from build123d import *

# Parameters (mm, degrees)
PAD_DEPTH       = 27.5
PAD_DEPTH_BACK  = 27.5
FILLET_R        = 2
SKETCH001_W     = 52
SKETCH001_H     = 11.986657
POCKET_DEPTH    = 30
SKETCH002_R     = 1.65
POCKET001_DEPTH = 14.114999
SKETCH003_R     = 1.65
POCKET002_DEPTH = 2.001
FILLET001_R     = 2.5


with BuildPart() as part:
    # Sketch → Pad (new body, two sides)
    with BuildSketch(Plane.YZ) as pad_sk:
        Polygon((0, 0), (15, 0), (0, 40), align=None)
    extrude(amount=PAD_DEPTH)
    extrude(pad_sk.sketch, amount=-PAD_DEPTH_BACK)

    # Fillet
    fillet_edges = [part.edges().sort_by_distance(p)[0] for p in [
        (0, 0, 40),
        (0, 15, 0),
    ]]
    fillet(fillet_edges, radius=FILLET_R)

    # Sketch001 (on DatumPlane) → Pocket (cut)
    with BuildSketch(Plane.XY.offset(32)):
        with Locations((0, 7.993328)):
            Rectangle(SKETCH001_W, SKETCH001_H)
    extrude(amount=-POCKET_DEPTH, mode=Mode.SUBTRACT)

    # Sketch002 (on Face4 of Pocket) → Pocket001 (cut, through all)
    with BuildSketch(Plane(origin=(0, 0, 0), x_dir=(0, 0, -1), z_dir=(0, -1, 0))):
        with Locations((-14.485332, 22.5)):
            Circle(SKETCH002_R)
        with Locations((-14.485332, -22.5)):
            Circle(SKETCH002_R)
    extrude(amount=-POCKET001_DEPTH, mode=Mode.SUBTRACT)

    # Sketch003 (on Face15 of Pocket001) → Pocket002 (cut, through all)
    with BuildSketch(Plane(origin=(0, 0, 2), x_dir=(0, -1, 0), z_dir=(0, 0, 1))):
        with Locations((-7.986657, 15)):
            Circle(SKETCH003_R)
        with Locations((-7.986657, -15)):
            Circle(SKETCH003_R)
    extrude(amount=-POCKET002_DEPTH, mode=Mode.SUBTRACT)

    # Fillet001
    fillet001_edges = [part.edges().sort_by_distance(p)[0] for p in [
        (0, 2, 2),
    ]]
    fillet(fillet001_edges, radius=FILLET001_R)


solid = part.part
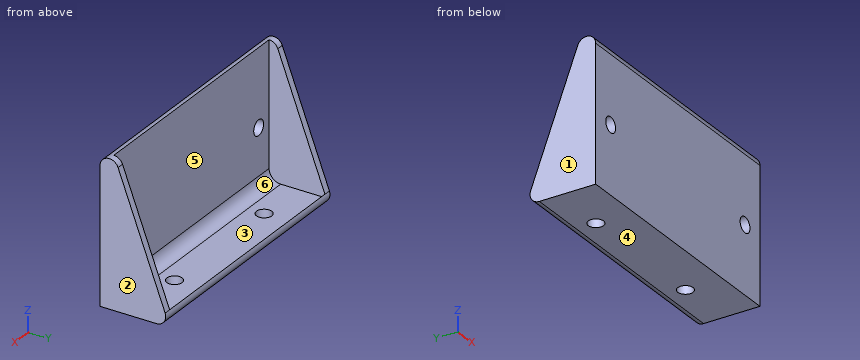
Can you work these out from the model? Positions are in its coordinate system, mm. Face numbers are marked on the shaded views. A direction names the side the tool comes from. Round coordinates to 2 decimals unless told otherwise and drop trailing zeros. Loops run counter-clockwise (first coordinate to the right, second up) from the corner with the lowest first, then second, coordinate; pieces in that order, holes last. Notation, with made-up numbers: (65.5, 7.25) - (115.5, 7.25) arc R26 cw to (115.5, 41.25) - close; hole circle Ø9 at (67, 28). An arc over 180 degrees is marked (long way). Use CSV: the item, a comma, the result in double quotes. Start each with the question number.
1) We'd pull the mould along X, two halves only. Please class the marked faces 1, 2 and 3: released by +X, released by -X, zero draft, split by the parting line, or undercut.
2) If we section it at B-B on y = 8.25: Write out the boundary of the cut face in (x, z).
3) For pin 1 Ø8 at (x, z) = (-7, 16) entering from +Y; pin 2 Ø3 at (x, z) = (22.5, 14.49) entering from -Y; pin 3 Ø1 at (x, y) = (-21, 11) entering from +Z; pin 4 Ø7.5 at (x, y) = (13, 7.5) entering from +Z, each with a flat end and sliding along its axis, tell me the tip position at first contact or that it passes through.
4) For the marked faces 4, 5 and 6, which set-ups out of +Z, -Z, +X, -X, +Y, -Y let a thin tool reach every point of the face, with its end or its side?
5) If we section it at C-C on z = 7: Write out the boundary of the cut face in (x, y) (3 decimals).
6) Please list where these lines run through material, in increasing order: probe 1 along X at (y, z) = (5.75, 15.5); probe 2 along Z at (x, y) = (-23.5, 6). Write a range as [from, to].
Geometry results:
1,face 1,"released by -X"
1,face 2,"released by +X"
1,face 3,"undercut"
2,outline,"(-27.5, 0) - (-16.63, 0) - (-16.63, 2) - (-26, 2) - (-26, 18) - (-27.5, 18) - close; (-13.37, 0) - (13.37, 0) - (13.37, 2) - (-13.37, 2) - close; (16.63, 0) - (27.5, 0) - (27.5, 18) - (26, 18) - (26, 2) - (16.63, 2) - close"
3,pin 1,"stops at y = 2"
3,pin 2,"passes through"
3,pin 3,"stops at z = 2"
3,pin 4,"stops at z = 2.12"
4,face 4,"-Z, +X, -X, +Y, -Y"
4,face 5,"+Z, +Y"
4,face 6,"+Z"
5,outline,"(-27.5, 0) - (27.5, 0) - (27.5, 12.375) - (26, 12.375) - (26, 2) - (-26, 2) - (-26, 12.375) - (-27.5, 12.375) - close"
6,probe 1,"x = [-27.5, -26], [26, 27.5]"
6,probe 2,"z = [0, 2]"
